```python
from build123d import *

# Parameters (mm, degrees)
SKETCH1_R               = 1.75
BOSS_EXTRUDE1_DEPTH     = 5
SKETCH2_W               = 10
SKETCH2_H               = 36
BOSS_EXTRUDE2_DEPTH     = 10.5
SKETCH3_R               = 1.75
BOSS_EXTRUDE3_DEPTH     = 5
FILLET1_R               = 5
SKETCH4_R               = 1.65
CUT_EXTRUDE1_DEPTH      = 43.444080859
SKETCH5_R               = 6.5
SKETCH5_R_2             = 2.5
BOSS_EXTRUDE4_DEPTH     = 11
BOSS_EXTRUDE5_START     = 5
BOSS_EXTRUDE5_DEPTH     = 5
CUT_EXTRUDE2_DEPTH      = 41.267853183
CUT_EXTRUDE2_DEPTH_BACK = 41.267853183
SKETCH7_R               = 1.75
FILLET2_R               = 5
FILLET3_R               = 5
SKETCH9_W               = 13.35
SKETCH9_H               = 12
BOSS_EXTRUDE6_DEPTH     = 10
CHAMFER2_SIZE           = 3
CHAMFER3_SIZE           = 3
FILLET6_R               = 2
SKETCH14_R              = 1.75
BOSS_EXTRUDE9_DEPTH     = 7
FILLET7_R               = 10
CUT_EXTRUDE7_DEPTH      = 52.802509666
CUT_EXTRUDE7_DEPTH_BACK = 52.802509666
CUT_EXTRUDE8_START      = -12
CUT_EXTRUDE8_DEPTH      = 12
SKETCH19_W              = 10
SKETCH19_H              = 15.5
BOSS_EXTRUDE10_DEPTH    = 10
BOSS_EXTRUDE11_START    = -27.5
BOSS_EXTRUDE11_DEPTH    = 27.5
CUT_EXTRUDE9_DEPTH      = 25
FILLET10_R              = 5


# Read off the part's stored shape, not the designer's step: Cut-Extrude8, Cut-Extrude9
with BuildPart() as part:
    # Sketch1 → Boss-Extrude1 (new body)
    with BuildSketch(Plane(origin=(0, 0, 0), x_dir=(1, 0, 0), z_dir=(0, 1, 0))):
        with BuildLine():
            Line((0, 5), (5.5, 5))
            Line((5.5, 5), (5.5, 31))
            Line((5.5, 31), (15.5, 31))
            Line((15.5, 31), (15.5, -5))
            Line((15.5, -5), (5.5, -5))
            Line((5.5, -5), (0, -5))
            ThreePointArc((0, -5), (-5, 0), (0, 5))
        make_face()
        with Locations(Location((0, 0, 0), (0, 0, 270))):
            Circle(SKETCH1_R, mode=Mode.SUBTRACT)
    extrude(amount=BOSS_EXTRUDE1_DEPTH)

    # Sketch2 → Boss-Extrude2 (add)
    with BuildSketch(Plane(origin=(0, 5, 0), x_dir=(1, 0, 0), z_dir=(0, 1, 0))):
        with Locations((10.5, 13)):
            Rectangle(SKETCH2_W, SKETCH2_H)
    extrude(amount=BOSS_EXTRUDE2_DEPTH)

    # Sketch3 → Boss-Extrude3 (add)
    with BuildSketch(Plane(origin=(0, 15.5, 0), x_dir=(1, 0, 0), z_dir=(0, 1, 0))):
        with BuildLine():
            Line((5.5, 5), (15.5, 5))
            Line((15.5, 5), (15.5, -5))
            Line((15.5, -5), (5.5, -5))
            Line((5.5, -5), (0, -5))
            ThreePointArc((0, -5), (-5, 0), (0, 5))
            Line((0, 5), (5.5, 5))
        make_face()
        with Locations(Location((0, 0, 0), (0, 0, 270))):
            Circle(SKETCH3_R, mode=Mode.SUBTRACT)
    extrude(amount=BOSS_EXTRUDE3_DEPTH)

    # Fillet1
    fillet1_edges = [part.edges().sort_by_distance(p)[0] for p in [
        (15.5, 10.25, 5),
    ]]
    fillet(fillet1_edges, radius=FILLET1_R)

    # Sketch4 → Cut-Extrude1 (cut, through all)
    with BuildSketch(Plane(origin=(15.5, 0, 0), x_dir=(0, 0, -1), z_dir=(1, 0, 0))):
        with Locations((20, 10.25)):
            Circle(SKETCH4_R)
    extrude(amount=-CUT_EXTRUDE1_DEPTH, mode=Mode.SUBTRACT)

    # Sketch5 → Boss-Extrude4 (add)
    with BuildSketch(Plane.XZ):
        with Locations(Location((5.5, -10, 0), (0, 0, 270))):
            Circle(SKETCH5_R)
        with Locations(Location((5.5, -10, 0), (0, 0, 270))):
            Circle(SKETCH5_R_2, mode=Mode.SUBTRACT)
    extrude(amount=BOSS_EXTRUDE4_DEPTH)

    # Sketch6 → Boss-Extrude5 (add)
    with BuildSketch(Plane(origin=(0, 0, 0), x_dir=(1, 0, 0), z_dir=(0, 1, 0)).offset(BOSS_EXTRUDE5_START)):
        with BuildLine():
            Line((5.5, 12.5), (5.5, 16.5))
            ThreePointArc((5.5, 16.5), (-0.61350963, 12.207940217), (1.346688069, 5))
            Line((1.346688069, 5), (5.5, 5))
            Line((5.5, 5), (5.5, 7.5))
            ThreePointArc((5.5, 7.5), (3, 10), (5.5, 12.5))
        make_face()
    extrude(amount=-BOSS_EXTRUDE5_DEPTH)

    # Sketch7 → Cut-Extrude2 (cut, two sides: drawn at the far end of the back side and taken through both)
    with BuildSketch(Plane(origin=(0, 0, 0), x_dir=(0, 0, -1), z_dir=(1, 0, 0)).offset(-CUT_EXTRUDE2_DEPTH_BACK)):
        with Locations((10, -6)):
            Circle(SKETCH7_R)
    extrude(amount=CUT_EXTRUDE2_DEPTH + CUT_EXTRUDE2_DEPTH_BACK, mode=Mode.SUBTRACT)

    # Fillet2
    fillet2_edges = [part.edges().sort_by_distance(p)[0] for p in [
        (10.5, 15.5, -31),
        (10.5, 0, -31),
    ]]
    fillet(fillet2_edges, radius=FILLET2_R)

    # Fillet3
    # the kernel refuses this fillet: 5 mm, written as the material it adds along each edge
    with BuildSketch(Plane(origin=(15.5, 15.5, -5), x_dir=(0, 0, -1), z_dir=(-1, 0, 0))) as fillet3_piece_1:
        with BuildLine():
            CenterArc((FILLET3_R, -FILLET3_R), FILLET3_R, 90, 90)
            Line((0, -FILLET3_R), (0, 0))
            Line((0, 0), (FILLET3_R, 0))
        make_face()
    extrude(amount=10)

    # Sketch9 → Boss-Extrude6 (add)
    with BuildSketch(Plane.ZY.offset(-5.5)):
        with Locations((-11.675, 21.5)):
            Rectangle(SKETCH9_W, SKETCH9_H)
    extrude(amount=-BOSS_EXTRUDE6_DEPTH)

    # Chamfer2
    chamfer2_edges = [part.edges().sort_by_distance(p)[0] for p in [
        (5.5, -11, -7.5),
    ]]
    chamfer(chamfer2_edges, length=CHAMFER2_SIZE)

    # Chamfer3
    # the kernel refuses this chamfer: 3 mm, written as the material it takes off along each edge
    with BuildSketch(Plane(origin=(5.5, 0, 0.215048964), x_dir=(-0.02749587661058649, 0.9996219169112968, 0), z_dir=(0, 0, -1))) as chamfer3_piece_1_section:
        Polygon((CHAMFER3_SIZE * 0.999621916911, CHAMFER3_SIZE * 0.0274958766106), (-CHAMFER3_SIZE * 0.0274958766106, CHAMFER3_SIZE * 0.999621916911), (0, 0), align=None)
    chamfer3_piece_1 = extrude(amount=20.430097928, mode=Mode.PRIVATE)
    chamfer3_piece_1 = chamfer3_piece_1 & Plane(origin=(5.5, 1.082097371, -10), x_dir=(0, 0, 1), z_dir=(0, 1, 0)) * Cylinder(2.5, 53, mode=Mode.PRIVATE)
    add(chamfer3_piece_1, mode=Mode.SUBTRACT)

    # Fillet6
    fillet6_edges = [part.edges().sort_by_distance(p)[0] for p in [
        (3, 5, -10),
    ]]
    fillet(fillet6_edges, radius=FILLET6_R)

    # Sketch14 → Boss-Extrude9 (add)
    with BuildSketch(Plane(origin=(0, 20.5, 0), x_dir=(1, 0, 0), z_dir=(0, 1, 0))):
        with BuildLine():
            Line((0, -5), (10.5, -5))
            ThreePointArc((10.5, -5), (14.035533906, -3.535533906), (15.5, 0))
            Line((15.5, 0), (15.5, 5))
            Line((15.5, 5), (5.5, 5))
            Line((5.5, 5), (0, 5))
            ThreePointArc((0, 5), (-5, 0), (0, -5))
        make_face()
        with Locations(Location((0, 0, 0), (0, 0, 270))):
            Circle(SKETCH14_R, mode=Mode.SUBTRACT)
    extrude(amount=BOSS_EXTRUDE9_DEPTH)

    # Fillet7
    # the kernel refuses this fillet: 10 mm, written as the material it adds along each edge
    with BuildSketch(Plane(origin=(1.346688069, 5, -5), x_dir=(-0.41939386698079784, 0, -0.9078043755891976), z_dir=(0, -1, 0))) as fillet7_piece_1:
        with BuildLine():
            CenterArc((9.89760177, -9.026713968), FILLET7_R, 115.488537073, 42.147981554)
            Line((0.649714482, -5.22190376), (-0.275074246, -4.841422739))
            ThreePointArc((-0.275074246, -4.841422739), (-0.343011659, -1.641923188), (-0.907804376, -0.419393867))
            Line((-0.907804376, -0.419393867), (0.430330512, 0.902671397))
            ThreePointArc((0.430330512, 0.902671397), (2.797148326, 0.367364079), (5.163966141, 0.902671397))
            Line((5.163966141, 0.902671397), (5.594296652, 0))
        make_face()
    extrude(amount=5)

    # Sketch17 → Cut-Extrude7 (cut, two sides: drawn at the far end of the back side and taken through both)
    with BuildSketch(Plane(origin=(0, 27.5, 0), x_dir=(1, 0, 0), z_dir=(0, 1, 0)).offset(-CUT_EXTRUDE7_DEPTH_BACK)):
        with BuildLine():
            Line((5.5, 3.5), (5.5, -5))
            Line((5.5, -5), (0, -5))
            ThreePointArc((0, -5), (-4.582515477, -2.000137971), (-3.666265283, 3.399779239))
            ThreePointArc((-3.666265283, 3.399779239), (-1.711748558, 6.491136994), (-0.999525638, 10.078526979))
            ThreePointArc((-0.999525638, 10.078526979), (0.876125793, 5.431653766), (5.5, 3.5))
        make_face()
    extrude(amount=CUT_EXTRUDE7_DEPTH + CUT_EXTRUDE7_DEPTH_BACK, mode=Mode.SUBTRACT)

    # Cut-Extrude8 outline → Cut-Extrude8 (cut)
    with BuildSketch(Plane.XZ.offset(-15.5).offset(CUT_EXTRUDE8_START)):
        with BuildLine():
            Line((1.346688069, -5), (5.5, -5))
            Line((5.5, -5), (5.5, -3.5))
            ThreePointArc((5.5, -3.5), (3.292059784, -3.88649037), (1.346688069, -5))
        make_face()
    extrude(amount=CUT_EXTRUDE8_DEPTH, mode=Mode.SUBTRACT)

    # Sketch19 → Boss-Extrude10 (add)
    with BuildSketch(Plane.ZY.offset(-5.5)):
        with Locations((10, 7.75)):
            Rectangle(SKETCH19_W, SKETCH19_H)
    extrude(amount=-BOSS_EXTRUDE10_DEPTH)

    # Sketch20 → Boss-Extrude11 (add)
    with BuildSketch(Plane.XZ.offset(BOSS_EXTRUDE11_START)):
        with BuildLine():
            Line((15.5, 5), (15.5, 0))
            ThreePointArc((15.5, 0), (14.035533906, 3.535533906), (10.5, 5))
            Line((10.5, 5), (15.5, 5))
        make_face()
    extrude(amount=BOSS_EXTRUDE11_DEPTH)

    # Cut-Extrude9 outline → Cut-Extrude9 (cut)
    with BuildSketch(Plane(origin=(0, 0, -10), x_dir=(0, 1, 0), z_dir=(0, 0, 1))):
        Polygon((5, 1), (-11, 1), (-11, -15.5), (27.5, -15.5), (27.5, -5.5), (5, -5.5), align=None)
    extrude(amount=CUT_EXTRUDE9_DEPTH, mode=Mode.SUBTRACT)

    # Fillet10
    fillet10_edges = [part.edges().sort_by_distance(p)[0] for p in [
        (10.5, 15.5, -18.35),
        (10.5, 27.5, -18.35),
    ]]
    fillet(fillet10_edges, radius=FILLET10_R)

    # Mirror1: part across plane


with BuildPart() as part_1:
    add(part.part)
    add(part.part.mirror(Plane.XY.offset(-10)))


solid = part_1.part
```
The listing builds one solid part. Answer for the finished solid, in the listing's coordinates (mm). A direction names the side the tool comes from. Give positions to 0.01 mm unless a question says otherwise; leave off trailing zeros. Order: outer loops, then holes, each group sorted by start corner. A loop starts at its lowest first (then second) coordinate and runs counter-clockwise, first axis right, second up. Notation, with made-up numbers: (30, 0.25) -> (48, 0.25) arc R12 ccw to (48, 21.25) -> close; hole circle Ø6 at (82, 43.25). An arc over 180 degrees is marked (long way). Answer as a JSON object with one key per item and string values. Group by question number.
Item 1: A tool of negligible diameter and unlimited length cuts with its end or side. For faces 5 (the flat face through (10, 8, -31)), 6 (the flat face through (10, 15.5, 5)), from which of +Z, -Z, +X, -X, +Y, -Y can it reach the whole face along a straight path? Write none if from no direction.
Item 2: Determine the mould class of faces 1 (the cylindrical face through (10.57, 8.64, -0.36)), 2 (the cylindrical face through (10.57, 9.25, -18.69)), 3 (the flat face through (15.5, 11, -10)), 4 (the flat face through (10, 21, -18.35)) for opening direction Z: pulls with the +Z half, pulls with the -Z half, needs draft (parallel to the pull), parting line crosses it, or undercut.
Item 3: The part is cut by section D-D on y = -2. Write down the section's boundary in (x, z).
Item 4: The part is cut by section A-A on z = 0. Write down the section's boundary in (x, y).
Item 5: The part is cut by section C-C on x = 8.5. Give the number of separate pieces and of enclosed holes in the cut face, and give its area (3 significant figures).
Item 6: Flat-ended cylindrical pins translate along their axes: pin 1 (0.8 mm diameter, centred on x = 10.5, z = -25, fed in from +Y); pin 2 (8 mm diameter, centred on x = 13, y = 23, fed in from -Z); pin 3 (1 mm diameter, centred on x = 8, z = -10, fed in from -Y). Find the tip coordinate at first contact, or state that the pin passes through.
Item 7: The part is cut by section B-B on y = -6. Write down the section's boundary in (x, z), and give its area (3 significant figures).
Item 8: Consider L1, parallel to X at y = 15.5, z = -11.5; L2, parallel to Y at x = 13, z = -20; L3, parallel to Z at x = 8.25, y = -9. Determine where each line is inside the solid, lowest interval first. Write a range as from..to.
Result set:
{
 "1": {"face 5": "-Z, +X, -X, +Y, -Y", "face 6": "+Z, +X, -X, +Y"},
 "2": {"face 1": "undercut", "face 2": "undercut", "face 3": "needs draft", "face 4": "pulls with the -Z half"},
 "3": {"outline": "circle Ø13 at (5.5, -10); hole circle Ø5 at (5.5, -10)"},
 "4": {"outline": "(5.5, 0) -> (15.5, 0) -> (15.5, 8.6) -> (5.5, 8.6) -> close; (5.5, 11.9) -> (15.5, 11.9) -> (15.5, 16.79) -> (5.5, 16.79) -> close"},
 "5": {"separate pieces": "1", "enclosed holes": "3", "area": "916 mm²"},
 "6": {"pin 1": "y = 15.5", "pin 2": "z = -18.58", "pin 3": "y = -8.5"},
 "7": {"outline": "(-0.76, -11.75) arc R6.5 ccw to (11.76, -11.75) -> (7.29, -11.75) arc R2.5 cw to (3.71, -11.75) -> close; (-0.76, -8.25) -> (3.71, -8.25) arc R2.5 cw to (7.29, -8.25) -> (11.76, -8.25) arc R6.5 ccw to start", "area": "84.1 mm²"},
 "8": {"L1": "5.5..15.5", "L2": "0..8.6, 11.9..16.79", "L3": "-15.89..-12.17, -7.83..-4.11"}
}
